from build123d import *

# Parameters (mm, degrees)
BOSS_EXTRU_2_DEPTH        = 5
ESQUISSE2_R               = 3
ENL_V_MAT_EXTRU_1_DEPTH   = 169.07736314
SYM_TRIE2_COPY_1_SKETCH_R = 3
SYM_TRIE2_COPY_1_DEPTH    = 169.07736314
ESQUISSE4_W               = 40
ESQUISSE4_H               = 37.5
ENL_V_MAT_EXTRU_2_DEPTH   = 60
ESQUISSE5_W               = 45
ESQUISSE5_H               = 5
BOSS_EXTRU_3_DEPTH        = 60
ESQUISSE7_W               = 230
ESQUISSE7_H               = 5
ENL_V_MAT_EXTRU_3_DEPTH   = 5
ESQUISSE11_W              = 15
ESQUISSE11_H              = 60
ENL_V_MAT_EXTRU_4_DEPTH   = 10
ESQUISSE12_W              = 5
ESQUISSE12_H              = 60
BOSS_EXTRU_4_DEPTH        = 5


with BuildPart() as part:
    # Esquisse1 → Boss.-Extru.2 (new body)
    with BuildSketch(Plane.XY):
        Polygon((135, 100), (-135, 100), (-135, 22.5), (-90, 22.5), (-90, -22.5), (-135, -22.5), (-135, -100), (135, -100), align=None)
    extrude(amount=BOSS_EXTRU_2_DEPTH)

    # Esquisse2 → Enlèv. mat.-Extru.1 (cut, through all)
    with BuildSketch(Plane.XY.offset(5)):
        with Locations((110, -75)):
            Circle(ESQUISSE2_R)
    enl_v_mat_extru_1 = extrude(amount=-ENL_V_MAT_EXTRU_1_DEPTH, mode=Mode.SUBTRACT)

    # Symétrie1: Enlèv. mat.-Extru.1 across plane
    add(enl_v_mat_extru_1.mirror(Plane(origin=(0, 0, 0), x_dir=(0, 0, 1), z_dir=(1, 0, 0))), mode=Mode.SUBTRACT)

    # Symétrie2: Enlèv. mat.-Extru.1 across plane
    add(enl_v_mat_extru_1.mirror(Plane(origin=(0, 0, 0), x_dir=(0, 0, 1), z_dir=(0, -1, 0))), mode=Mode.SUBTRACT)

    # Symétrie2 copy 1 sketch → Symétrie2 copy 1 (cut, through all)
    with BuildSketch(Plane(origin=(0, 0, 5), x_dir=(-1, 0, 0), z_dir=(0, 0, 1))):
        with Locations((110, -75)):
            Circle(SYM_TRIE2_COPY_1_SKETCH_R)
    extrude(amount=-SYM_TRIE2_COPY_1_DEPTH, mode=Mode.SUBTRACT)

    # Esquisse4 → Enlèv. mat.-Extru.2 (cut)
    with BuildSketch(Plane.XY.offset(5)):
        with Locations((-102.5, -76.25)):
            Rectangle(ESQUISSE4_W, ESQUISSE4_H)
    extrude(amount=-ENL_V_MAT_EXTRU_2_DEPTH, mode=Mode.SUBTRACT)

    # Esquisse5 → Boss.-Extru.3 (add)
    with BuildSketch(Plane(origin=(0, -22.5, 0), x_dir=(1, 0, 0), z_dir=(0, 1, 0))):
        with Locations((-112.5, -2.5)):
            Rectangle(ESQUISSE5_W, ESQUISSE5_H)
    extrude(amount=BOSS_EXTRU_3_DEPTH)

    # Esquisse7 → Enlèv. mat.-Extru.3 (cut)
    with BuildSketch(Plane(origin=(0, 100, 0), x_dir=(1, 0, 0), z_dir=(0, 1, 0))):
        with Locations((0, -2.5)):
            Rectangle(ESQUISSE7_W, ESQUISSE7_H)
    extrude(amount=-ENL_V_MAT_EXTRU_3_DEPTH, mode=Mode.SUBTRACT)

    # Esquisse11 → Enlèv. mat.-Extru.4 (cut)
    with BuildSketch(Plane(origin=(0, 0, 0), x_dir=(-1, 0, 0), z_dir=(0, 0, -1))):
        with Locations((0, 65)):
            Rectangle(ESQUISSE11_W, ESQUISSE11_H)
    extrude(amount=-ENL_V_MAT_EXTRU_4_DEPTH, mode=Mode.SUBTRACT)

    # Esquisse12 → Boss.-Extru.4 (add)
    with BuildSketch(Plane.ZY.offset(-7.5)):
        with Locations((2.5, 65)):
            Rectangle(ESQUISSE12_W, ESQUISSE12_H)
    extrude(amount=BOSS_EXTRU_4_DEPTH)


solid = part.part
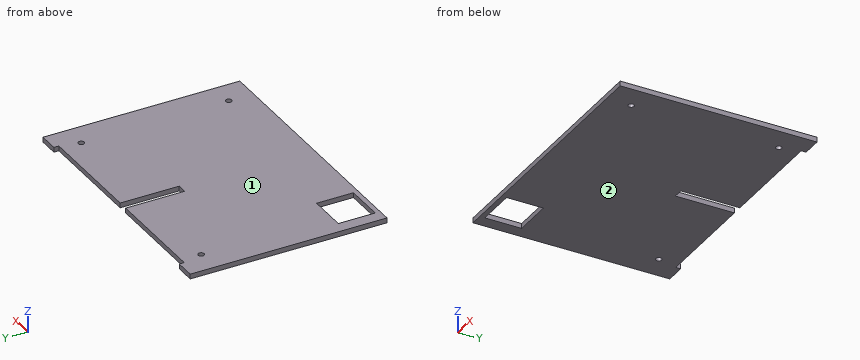
Verification items for the finished model (mm, model axes). Face numbers are marked on the shaded views. Round coordinates to 2 decimals unless told otherwise and drop trailing zeros. Loops run counter-clockwise (first coordinate to the right, second up) from the corner with the lowest first, then second, coordinate; pieces in that order, holes last. Notation, with made-up numbers: (76.5, -31.5) - (92.5, -31.5) arc R28 cw to (92.5, 3.5) - close; hole circle Ø8 at (66.25, 43.5). An arc over 180 degrees is marked (long way). Answer in a Markdown table with one row per item. Add a question column.
Q1. Release check for a two-part mould opening along Z. For the marked faces 1 and 2 record: pulls with the +Z half, pulls with the -Z half, needs draft (parallel to the pull), parting line crosses it, or undercut.
Q2. Section check D-D on y = 75. Enter the section's corners in (x, z).
Q3. Gauge pin test, flat ends, axial feed: pin 1 (3.5 mm diameter, centred on x = 110, y = 75, fed in from -Z); pin 2 (1.5 mm diameter, centred on x = -37, z = 3, fed in from +Y). Record the tip position at first contact, or that the pin passes through.
Q4. Section check C-C on z = 2.4. Enter the section's corners in (x, y).
Q5. Material ranges on line 1 (X direction, y = 75, z = 2.6); line 2 (Y direction, x = 110, z = 3); line 3 (Y direction, x = -110, z = 2.1), recorded low to high.
Q6. Section check A-A on y = 42. Enter the section's corners in (x, z), plus the area to 3 significant figures.
Q7. Section check B-B on x = 110. Enter the section's corners in (y, z).
Found:
| question | item | result |
|---|---|---|
| 1 | face 1 | pulls with the +Z half |
| 1 | face 2 | pulls with the -Z half |
| 2 | outline | (-135, 0) - (-113, 0) - (-113, 5) - (-135, 5) - close; (-107, 0) - (-7.5, 0) - (-7.5, 5) - (-107, 5) - close; (2.5, 0) - (107, 0) - (107, 5) - (2.5, 5) - close; (113, 0) - (135, 0) - (135, 5) - (113, 5) - close |
| 3 | pin 1 | passes through |
| 3 | pin 2 | stops at y = 95 |
| 4 | outline | (-135, -100) - (135, -100) - (135, 100) - (115, 100) - (115, 95) - (2.5, 95) - (2.5, 35) - (-7.5, 35) - (-7.5, 95) - (-115, 95) - (-115, 100) - (-135, 100) - close; hole (-122.5, -95) - (-82.5, -95) - (-82.5, -57.5) - (-122.5, -57.5) - close; hole circle Ø6 at (-110, 75); hole circle Ø6 at (110, -75); hole circle Ø6 at (110, 75) |
| 5 | line 1 | x = -135 to -113, -107 to -7.5, 2.5 to 107, 113 to 135 |
| 5 | line 2 | y = -100 to -78, -72 to 72, 78 to 95 |
| 5 | line 3 | y = -100 to -95, -57.5 to 72, 78 to 95 |
| 6 | outline | (-135, 0) - (-7.5, 0) - (-7.5, 5) - (-135, 5) - close; (2.5, 0) - (135, 0) - (135, 5) - (2.5, 5) - close |
| 6 | area | 1,300 mm² |
| 7 | outline | (-100, 0) - (-78, 0) - (-78, 5) - (-100, 5) - close; (-72, 0) - (72, 0) - (72, 5) - (-72, 5) - close; (78, 0) - (95, 0) - (95, 5) - (78, 5) - close |
